For this review, take the finished solid that the model builds, in its own axes (mm). A direction names the side the tool comes from. Coordinates: 2 decimals unless noted, no trailing zeros. Loops run counter-clockwise (first coordinate to the right, second up) from the corner with the lowest first, then second, coordinate; pieces in that order, holes last. Notation, with made-up numbers: (-36, 50) - (-20, 50) arc R26 ccw to (-20, 86) - close; hole circle Ø9 at (64.5, 31.5). An arc over 180 degrees is marked (long way). Answer as a JSON object with one key per item and string values. Group by question number.
Item 1: Mouldability with a two-part tool opening along X and no side actions: class faces 4 (the flat face through (21.5, -4, 2)), 5 (the cylindrical face through (-48.05, 8.18, 1.52)), 6 (the flat face through (-2, 14, 1)) as released by +X, released by -X, zero draft, split by the parting line, or undercut.
Item 2: We need section A-A (y = -53). Give the boundary of the cut face in (x, z).
Item 3: Clearance check with flat-ended pins moving along their axes: pin 1 (1 mm diameter, centred on x = -51, z = 1, fed in from -Y); pin 2 (1.5 mm diameter, centred on y = -7.5, z = 1, fed in from -X); pin 3 (1.5 mm diameter, centred on x = 4.5, z = 2, fed in from -Y). State where each tip first meets the part, or that it passes through.
Item 4: We need section B-B (z = 2.25). State how many separate pieces and enclosed holes the cut face has, then the cut area to 3 significant figures.
Item 5: Tool access review of faces 1 (the flat face through (24, -14, 1)), 2 (the flat face through (-53.06, -66.13, 1.52)), 3 (the flat face through (-61, -104, 1)): name each direction out of +Z, -Z, +X, -X, +Y, -Y from which nothing blocks a thin tool from reaching the whole face with its end or side.
Item 6: We need section C-C (x = -15.5). Give the boundary of the cut face in (y, z).
Item 7: To check wall thickness, follow line 1 (Y direction, x = 26, z = 0.65); line 2 (X direction, y = 0, z = 1.8); line 3 (X direction, y = -101.5, z = 0.95). State the ranges of each line that lie inside material, in increasing order.
from build123d import *

# Parameters (mm, degrees)
BOSS_EXTRU_1_DEPTH      = 3
ENL_V_MAT_EXTRU_1_REACH = 128.289
ESQUISSE2_W             = 40.2
ESQUISSE2_H             = 20.4
ENL_V_MAT_EXTRU_2_REACH = 128.289
ESQUISSE3_R             = 1.45
CONG_2_R                = 4.7
CONG_3_R                = 10
CONG_4_R                = 30
CONG_5_R                = 3.75
ENL_V_MAT_EXTRU_3_REACH = 128.289
CONG_6_R                = 1.5
ENL_V_MAT_EXTRU_4_REACH = 128.289
ESQUISSE5_R             = 1.15
ESQUISSE6_R             = 1.15
ENL_V_MAT_EXTRU_5_DEPTH = 10


with BuildPart() as part:
    # Esquisse1 → Boss.-Extru.1 (new body)
    with BuildSketch(Plane.XY):
        with BuildLine():
            Line((-30.9, 14), (-50.9, 14))
            ThreePointArc((-50.9, 14), (-68.065443638, -43.785518027), (-70.9, -104))
            Line((-70.9, -104), (-50.9, -104))
            ThreePointArc((-50.9, -104), (-45.084672315, -58.070072819), (-30.9, -14))
            Line((-30.9, -14), (30.9, -14))
            Line((30.9, -14), (30.9, 14))
            Line((30.9, 14), (-30.9, 14))
        make_face()
    extrude(amount=BOSS_EXTRU_1_DEPTH)

    # Esquisse2 → Enlèv. mat.-Extru.1 (cut, up to next)
    with BuildSketch(Plane.XY.offset(3), mode=Mode.PRIVATE) as enl_v_mat_extru_1_sk1:
        with Locations((1.4, -3.8)):
            Rectangle(ESQUISSE2_W, ESQUISSE2_H)
    enl_v_mat_extru_1_tool1 = extrude(enl_v_mat_extru_1_sk1.sketch, amount=-ENL_V_MAT_EXTRU_1_REACH, mode=Mode.PRIVATE) & part.part
    add(enl_v_mat_extru_1_tool1.solids().sort_by_distance((1.4, -3.8, 3))[0], mode=Mode.SUBTRACT)

    # Esquisse3 → Enlèv. mat.-Extru.2 (cut, up to next)
    with BuildSketch(Plane.XY.offset(3), mode=Mode.PRIVATE) as enl_v_mat_extru_2_sk1:
        with Locations((26.2, -8.8)):
            Circle(ESQUISSE3_R)
    enl_v_mat_extru_2_tool1 = extrude(enl_v_mat_extru_2_sk1.sketch, amount=-ENL_V_MAT_EXTRU_2_REACH, mode=Mode.PRIVATE) & part.part
    # Esquisse3 → Enlèv. mat.-Extru.2 (cut, up to next)
    with BuildSketch(Plane.XY.offset(3), mode=Mode.PRIVATE) as enl_v_mat_extru_2_sk2:
        with Locations((-23.4, -8.8)):
            Circle(ESQUISSE3_R)
    enl_v_mat_extru_2_tool2 = extrude(enl_v_mat_extru_2_sk2.sketch, amount=-ENL_V_MAT_EXTRU_2_REACH, mode=Mode.PRIVATE) & part.part
    # Esquisse3 → Enlèv. mat.-Extru.2 (cut, up to next)
    with BuildSketch(Plane.XY.offset(3), mode=Mode.PRIVATE) as enl_v_mat_extru_2_sk3:
        with Locations((-23.4, 1.2)):
            Circle(ESQUISSE3_R)
    enl_v_mat_extru_2_tool3 = extrude(enl_v_mat_extru_2_sk3.sketch, amount=-ENL_V_MAT_EXTRU_2_REACH, mode=Mode.PRIVATE) & part.part
    # Esquisse3 → Enlèv. mat.-Extru.2 (cut, up to next)
    with BuildSketch(Plane.XY.offset(3), mode=Mode.PRIVATE) as enl_v_mat_extru_2_sk4:
        with Locations((26.2, 1.2)):
            Circle(ESQUISSE3_R)
    enl_v_mat_extru_2_tool4 = extrude(enl_v_mat_extru_2_sk4.sketch, amount=-ENL_V_MAT_EXTRU_2_REACH, mode=Mode.PRIVATE) & part.part
    add(enl_v_mat_extru_2_tool1.solids().sort_by_distance((26.2, -8.8, 3))[0], mode=Mode.SUBTRACT)
    add(enl_v_mat_extru_2_tool2.solids().sort_by_distance((-23.4, -8.8, 3))[0], mode=Mode.SUBTRACT)
    add(enl_v_mat_extru_2_tool3.solids().sort_by_distance((-23.4, 1.2, 3))[0], mode=Mode.SUBTRACT)
    add(enl_v_mat_extru_2_tool4.solids().sort_by_distance((26.2, 1.2, 3))[0], mode=Mode.SUBTRACT)

    # Congé2
    cong_2_edges = [part.edges().sort_by_distance(p)[0] for p in [
        (30.9, -14, 1.5),
        (30.9, 14, 1.5),
    ]]
    fillet(cong_2_edges, radius=CONG_2_R)

    # Congé3
    cong_3_edges = [part.edges().sort_by_distance(p)[0] for p in [
        (-30.9, -14, 1.5),
    ]]
    fillet(cong_3_edges, radius=CONG_3_R)

    # Congé4
    cong_4_edges = [part.edges().sort_by_distance(p)[0] for p in [
        (-50.9, 14, 1.5),
    ]]
    fillet(cong_4_edges, radius=CONG_4_R)

    # Congé5
    cong_5_edges = [part.edges().sort_by_distance(p)[0] for p in [
        (-50.9, -104, 1.5),
        (-70.9, -104, 1.5),
    ]]
    fillet(cong_5_edges, radius=CONG_5_R)

    # Esquisse4 → Enlèv. mat.-Extru.3 (cut, up to next)
    with BuildSketch(Plane.XY.offset(3), mode=Mode.PRIVATE) as enl_v_mat_extru_3_sk1:
        Polygon((-33.484388558, -11.358463284), (-43.05887194, -28.83955138), (-50.238359759, -1.41390105), align=None)
    enl_v_mat_extru_3_tool1 = extrude(enl_v_mat_extru_3_sk1.sketch, amount=-ENL_V_MAT_EXTRU_3_REACH, mode=Mode.PRIVATE) & part.part
    # Esquisse4 → Enlèv. mat.-Extru.3 (cut, up to next)
    with BuildSketch(Plane.XY.offset(3), mode=Mode.PRIVATE) as enl_v_mat_extru_3_sk2:
        Polygon((-54.025759835, -8.664001443), (-47.704691317, -32.810489222), (-62.900626013, -49.913479621), align=None)
    enl_v_mat_extru_3_tool2 = extrude(enl_v_mat_extru_3_sk2.sketch, amount=-ENL_V_MAT_EXTRU_3_REACH, mode=Mode.PRIVATE) & part.part
    # Esquisse4 → Enlèv. mat.-Extru.3 (cut, up to next)
    with BuildSketch(Plane.XY.offset(3), mode=Mode.PRIVATE) as enl_v_mat_extru_3_sk3:
        Polygon((-44.434019708, -37.409998289), (-63.702500518, -59.0966302), (-62.097933842, -96.225533823), align=None)
    enl_v_mat_extru_3_tool3 = extrude(enl_v_mat_extru_3_sk3.sketch, amount=-ENL_V_MAT_EXTRU_3_REACH, mode=Mode.PRIVATE) & part.part
    # Esquisse4 → Enlèv. mat.-Extru.3 (cut, up to next)
    with BuildSketch(Plane.XY.offset(3), mode=Mode.PRIVATE) as enl_v_mat_extru_3_sk4:
        Polygon((-46.457316631, 3.078230456), (-30.208699652, -6.566371461), (-30.208699652, 9.392706582), align=None)
    enl_v_mat_extru_3_tool4 = extrude(enl_v_mat_extru_3_sk4.sketch, amount=-ENL_V_MAT_EXTRU_3_REACH, mode=Mode.PRIVATE) & part.part
    add(enl_v_mat_extru_3_tool1.solids().sort_by_distance((-42.26054, -13.870639, 3))[0], mode=Mode.SUBTRACT)
    add(enl_v_mat_extru_3_tool2.solids().sort_by_distance((-54.877026, -30.462657, 3))[0], mode=Mode.SUBTRACT)
    add(enl_v_mat_extru_3_tool3.solids().sort_by_distance((-56.744818, -64.244054, 3))[0], mode=Mode.SUBTRACT)
    add(enl_v_mat_extru_3_tool4.solids().sort_by_distance((-35.624905, 1.968189, 3))[0], mode=Mode.SUBTRACT)

    # Congé6
    cong_6_edges = [part.edges().sort_by_distance(p)[0] for p in [
        (-62.900626013, -49.913479621, 1.5),
        (-54.025759835, -8.664001443, 1.5),
        (-47.704691317, -32.810489222, 1.5),
        (-46.457316631, 3.078230456, 1.5),
        (-30.208699652, 9.392706582, 1.5),
        (-30.208699652, -6.566371461, 1.5),
        (-44.434019708, -37.409998289, 1.5),
        (-62.097933842, -96.225533823, 1.5),
        (-63.702500518, -59.0966302, 1.5),
        (-50.238359759, -1.41390105, 1.5),
        (-33.484388558, -11.358463284, 1.5),
        (-43.05887194, -28.83955138, 1.5),
    ]]
    fillet(cong_6_edges, radius=CONG_6_R)

    # Esquisse5 → Enlèv. mat.-Extru.4 (cut, up to next)
    with BuildSketch(Plane.XY.offset(3), mode=Mode.PRIVATE) as enl_v_mat_extru_4_sk1:
        with Locations((16.4, 8.9)):
            Circle(ESQUISSE5_R)
    enl_v_mat_extru_4_tool1 = extrude(enl_v_mat_extru_4_sk1.sketch, amount=-ENL_V_MAT_EXTRU_4_REACH, mode=Mode.PRIVATE) & part.part
    # Esquisse5 → Enlèv. mat.-Extru.4 (cut, up to next)
    with BuildSketch(Plane.XY.offset(3), mode=Mode.PRIVATE) as enl_v_mat_extru_4_sk2:
        with Locations((6.4, 8.9)):
            Circle(ESQUISSE5_R)
    enl_v_mat_extru_4_tool2 = extrude(enl_v_mat_extru_4_sk2.sketch, amount=-ENL_V_MAT_EXTRU_4_REACH, mode=Mode.PRIVATE) & part.part
    add(enl_v_mat_extru_4_tool1.solids().sort_by_distance((16.4, 8.9, 3))[0], mode=Mode.SUBTRACT)
    add(enl_v_mat_extru_4_tool2.solids().sort_by_distance((6.4, 8.9, 3))[0], mode=Mode.SUBTRACT)

    # Esquisse6 → Enlèv. mat.-Extru.5 (cut)
    with BuildSketch(Plane.XY.offset(3)):
        with Locations((-65.945726783, -101.5)):
            Circle(ESQUISSE6_R)
        with Locations((-55.945726783, -101.5)):
            Circle(ESQUISSE6_R)
    extrude(amount=-ENL_V_MAT_EXTRU_5_DEPTH, mode=Mode.SUBTRACT)


solid = part.part
Check sheet entries:
{
 "1": {"face 4": "undercut", "face 5": "released by -X", "face 6": "zero draft"},
 "2": {"outline": "(-69.45, 0) - (-58.29, 0) - (-58.29, 3) - (-69.45, 3) - close; (-49.12, 0) - (-43.9, 0) - (-43.9, 3) - (-49.12, 3) - close"},
 "3": {"pin 1": "stops at y = -102.5", "pin 2": "stops at x = -59.33", "pin 3": "stops at y = 6.4"},
 "4": {"separate pieces": "1", "enclosed holes": "12", "area": "2,840 mm2"},
 "5": {"face 1": "+Z, -Z, +X, -Y", "face 2": "+Z, -Z", "face 3": "+Z, -Z, +X, -X, -Y"},
 "6": {"outline": "(6.4, 0) - (14, 0) - (14, 3) - (6.4, 3) - close"},
 "7": {"line 1": "y = -14 to -10.24, -7.36 to -0.24, 2.64 to 14", "line 2": "x = -55.67 to -41.27, -30.21 to -24.21, -22.59 to -18.7, 21.5 to 25.39, 27.01 to 30.9", "line 3": "x = -70.93 to -67.1, -64.8 to -57.1, -54.8 to -50.97"}
}
